Part print with two shaded views. Sizes in mm from the minimum x, y, z corner. A direction names the side the tool comes from. Round coordinates to 2 decimals unless told otherwise and drop trailing zeros. Order: outer loops, then holes, each group sorted by start corner. A loop starts at its lowest first (then second) coordinate and runs counter-clockwise, first axis right, second up. Notation, with made-up numbers: (-2, 66) - (18, 66) arc R18 ccw to (18, 78) - close; hole circle Ø6 at (-1, -16). An arc over 180 degrees is marked (long way). Write item = value, one per line.
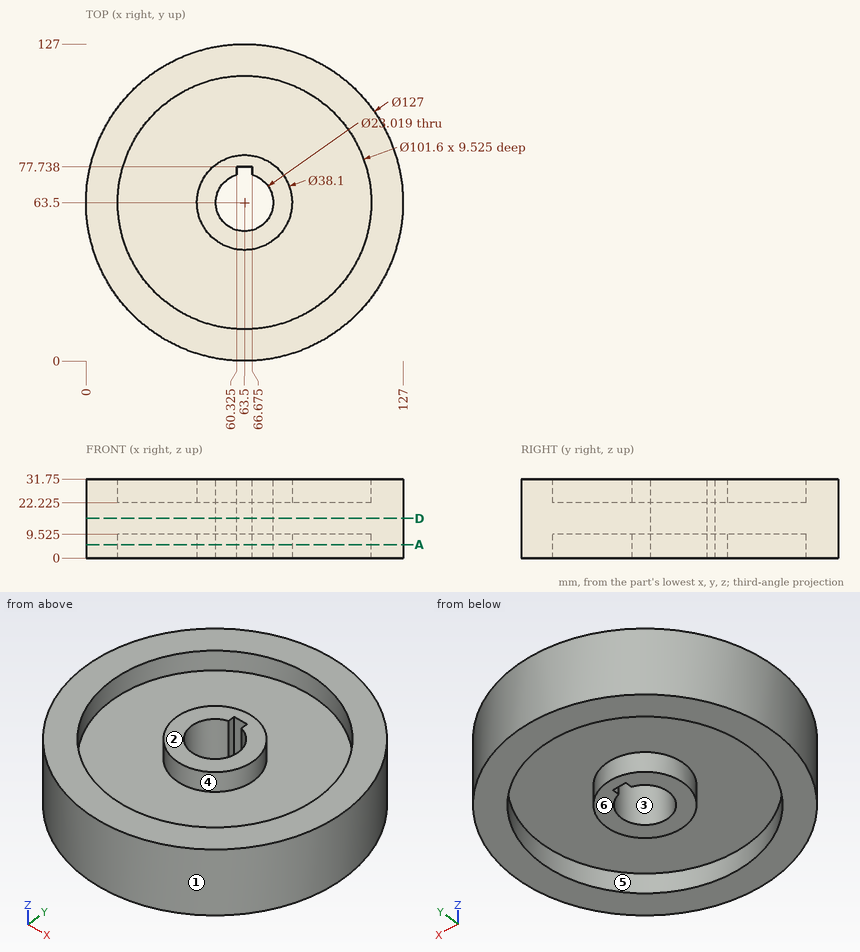
1) Flat gauge pins, fed straight in: pin 1 Ø8 at (y, z) = (83.5, 16) entering from -X; pin 2 Ø8 at (x, y) = (25.5, 86) entering from +Z (3 decimals); pin 3 Ø3.5 at (y, z) = (76, 13.5) entering from -X. Where does each tip first touch, or does it go through?
Conclusion:
pin_1 = 2.05
pin_2 = 22.225
pin_3 = 0.92
2) Mould opens along X. For the marked faces 1, 2 and 3 say: +X half, -X half, draft (parallel to the pull), parting line (faces both ways), or undercut.
Conclusion:
face_1 = parting line
face_2 = draft
face_3 = undercut
3) Cut at A-A (z = 5.5). Give the number of separate pieces and of enclosed holes in the cut face, and give its area (3 significant figures).
Conclusion:
separate_pieces = 2
enclosed_holes = 2
area = 5,270 mm^2
4) 3-axis set-ups, long thin cutter, end or side, ignore diameter. For the marked faces 4, 5 and 6: which of +Z, -Z, +X, -X, +Y, -Y reach the whole face in a straight line?
Conclusion:
face_4 = +Z
face_5 = -Z
face_6 = -Z, +X, -X, +Y, -Y
5) Wall check: line 1 along X through (y, z) = (63.5, 5.25); line 2 along Y through (x, z) = (63, 20); line 3 along X through (y, z) = (63.5, 21.5). Give the ranges that are in metal, low to high.
Conclusion:
line_1 = 0 to 12.7, 44.45 to 51.99, 75.01 to 82.55, 114.3 to 127
line_2 = 0 to 52, 77.74 to 127
line_3 = 0 to 51.99, 75.01 to 127
6) Cut at D-D (z = 16). Write the cut outline in (x, y) (1 decimal).
Conclusion:
outline = circle Ø127 at (63.5, 63.5); hole (60.3, 74.6) arc R11.5 ccw (long way) to (66.7, 74.6) - (66.7, 77.7) - (60.3, 77.7) - close
